Could you check a few things on this drawing? It's one solid part, dimensions in mm from its lowest x, y, z. A direction names the side the tool comes from. Coordinates: 2 decimals unless noted, no trailing zeros. Order: outer loops, then holes, each group sorted by start corner. A loop starts at its lowest first (then second) coordinate and runs counter-clockwise, first axis right, second up. Notation, with made-up numbers: M 16.5,-32.75 L 20.5,-32.75 A20 cw 20.5,-25.75 Z; hole C -29.75,86 d9. An arc over 180 degrees is marked long. Answer as CSV lines item,"result". Start each with the question number.
1. I need wall thicknesses on line 1 along X through (y, z) = (12.5, 1.75); line 2 along Y through (x, z) = (37.5, 9); line 3 along X through (y, z) = (23, 22). Which ranges of each line are inside material? Lowest first, please. Write a range as from..to.
2. If we section it at D-D (x = 31): List the corners of the cut face in (y, z) for me.
3. If we section it at C-C (y = 4): List the corners of the cut face in (x, z) for me.
4. If we section it at A-A (y = 23.5): List the corners of the cut face in (x, z) for me, plus the area to 3 significant figures.
5. Will this pin go through, and if not, where does the flat tip stop? pin 1 (12 mm diameter, centred on x = 43, y = 8.5, fed in from +Z).
6. If we mould it in two halves opening along X, with no side actions, what happens to the marked faces 3, 4, 5 and 6? For each: released by +X, released by -X, zero draft, split by the parting line, or undercut.
7. If we section it at B-B (z = 24.25): List the corners of the cut face in (x, y) for me.
8. On a 3-axis mill with a long thin cutter (end or side, diameter ignored), from which of +Z, -Z, +X, -X, +Y, -Y can I reach the whole of each face in a straight line? I mean the marked faces 1 and 2. Say none if no direction works.
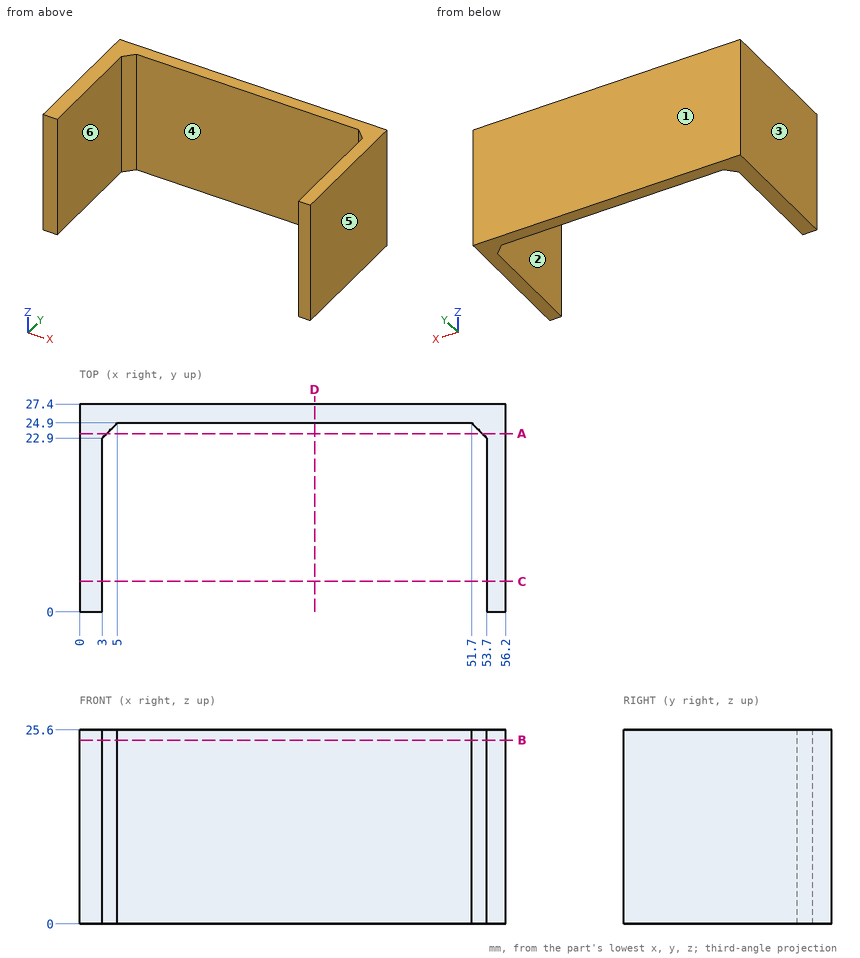
Solved:
1,line 1,"0..3, 53.7..56.2"
1,line 2,"24.9..27.4"
1,line 3,"0..3.1, 53.6..56.2"
2,outline,"M 24.9,0 L 27.4,0 L 27.4,25.6 L 24.9,25.6 Z"
3,outline,"M 0,0 L 3,0 L 3,25.6 L 0,25.6 Z; M 53.7,0 L 56.2,0 L 56.2,25.6 L 53.7,25.6 Z"
4,outline,"M 0,0 L 3.6,0 L 3.6,25.6 L 0,25.6 Z; M 53.1,0 L 56.2,0 L 56.2,25.6 L 53.1,25.6 Z"
4,area,"172 mm²"
5,pin 1,"through"
6,face 3,"released by -X"
6,face 4,"undercut"
6,face 5,"released by +X"
6,face 6,"undercut"
7,outline,"M 0,0 L 3,0 L 3,22.9 L 5,24.9 L 51.7,24.9 L 53.7,22.9 L 53.7,0 L 56.2,0 L 56.2,27.4 L 0,27.4 Z"
8,face 1,"+Z, -Z, +X, -X, +Y"
8,face 2,"+Z, -Z, -Y"
